from build123d import *

# Parameters (mm, degrees)
SKETCH_1_W          = 7.2
SKETCH_1_H          = 5
EXTRUDE_1_DEPTH     = 1.2
SKETCH_2_R          = 1.85
CUT_EXTRUDE_1_DEPTH = 5.544227107
SKETCH_3_W          = 1.2
SKETCH_3_H          = 5
EXTRUDE_2_DEPTH     = 24
FILLET_1_R          = 0.3
SKETCH_4_R          = 2.05
CUT_EXTRUDE_2_DEPTH = 27.024795869
EXTRUDE_START       = 2
EXTRUDE_4_DEPTH     = 2
EXTRUDE_5_DEPTH     = 1.2


with BuildPart() as part:
    # 스케치1 → 보스-돌출1 (new body)
    with BuildSketch(Plane.XY):
        Rectangle(SKETCH_1_W, SKETCH_1_H)
    extrude(amount=EXTRUDE_1_DEPTH)

    # 스케치2 → 컷-돌출1 (cut, through all)
    with BuildSketch(Plane.XY.offset(1.2)):
        with Locations((-0.75, 0)):
            Circle(SKETCH_2_R)
    extrude(amount=-CUT_EXTRUDE_1_DEPTH, mode=Mode.SUBTRACT)

    # 스케치3 → 보스-돌출2 (add)
    with BuildSketch(Plane.XY.offset(1.2)):
        with Locations((3, 0)):
            Rectangle(SKETCH_3_W, SKETCH_3_H)
    extrude(amount=EXTRUDE_2_DEPTH)

    # 필렛1
    fillet_1_edges = [part.edges().sort_by_distance(p)[0] for p in [
        (2.4, 0, 1.2),
    ]]
    fillet(fillet_1_edges, radius=FILLET_1_R)

    # 스케치4 → 컷-돌출2 (cut, through all)
    with BuildSketch(Plane.ZY.offset(-2.4)):
        with Locations(Location((21.2, 0, 0), (0, 0, 270))):
            Circle(SKETCH_4_R)
        with Locations(Location((9.2, 0, 0), (0, 0, 270))):
            Circle(SKETCH_4_R)
    extrude(amount=-CUT_EXTRUDE_2_DEPTH, mode=Mode.SUBTRACT)

    # 스케치6 → 보스-돌출4 (add)
    with BuildSketch(Plane.XZ.offset(2.5).offset(EXTRUDE_START)):
        with BuildLine():
            Line((-3.6, 1.2), (-3.6, 0))
            Line((-3.6, 0), (3.6, 0))
            Line((3.6, 0), (3.6, 25.2))
            Line((3.6, 25.2), (2.4, 25.2))
            Line((2.4, 25.2), (2.4, 1.5))
            ThreePointArc((2.4, 1.5), (2.312132034, 1.287867966), (2.1, 1.2))
            Line((2.1, 1.2), (-3.6, 1.2))
        make_face()
    extrude_4 = extrude(amount=-EXTRUDE_4_DEPTH)

    # 대칭 복사1: 보스-돌출4 across plane
    add(extrude_4.mirror(Plane.ZX))

    # 스케치7 → 보스-돌출5 (add)
    with BuildSketch(Plane(origin=(0, -4.5, 0), x_dir=(-1, 0, 0), z_dir=(0, -1, 0))):
        Polygon((3.6, 0), (-3.6, 0), (-3.6, -25.2), (-2.4, -25.2), (3.6, -1.2), align=None)
    extrude_5 = extrude(amount=EXTRUDE_5_DEPTH)

    # 대칭 복사2: 보스-돌출5 across plane
    add(extrude_5.mirror(Plane.ZX))


solid = part.part
Design review of the part built by this model. Coordinates are the model's own, in mm. A direction names the side the tool comes from. Give positions to 0.01 mm unless a question says otherwise; leave off trailing zeros. Loops run counter-clockwise (first coordinate to the right, second up) from the corner with the lowest first, then second, coordinate; pieces in that order, holes last. Notation, with made-up numbers: (-4.5, -35.75) - (41.5, -35.75) arc R16 cw to (41.5, -9.75) - close; hole circle Ø7 at (-31.5, 3.5). An arc over 180 degrees is marked (long way). Use CSV: the item, a comma, the result in double quotes. Start each with the question number.
1. Insertion check: P1, Ø4.5, axis at y = 2, z = 18.5, coming from the -X side; P2, Ø4, axis at x = -1, z = 18, coming from the +Y side. Each pin has a flat end and moves straight along its axis. Give the tip position at first contact, or say it passes through.
2. Add section B-B (z = 21.2). State the section outline as (x, y) points.
3. Add section A-A (x = -0.75). State the section outline as (y, z) points.
4. Draft analysis for pull direction Y (two halves, no side actions). For faces 3 (the flat face through (1, -1, 0)), 4 (the cylindrical face through (2.992, 0.444, 19.199)), 5 (the flat face through (1, -5.7, 10)), 6 (the cylindrical face through (2.992, -0.946, 7.381)), state which applies: released by +Y, released by -Y, zero draft, split by the parting line, or undercut.
5. Wall thickness on L1, parallel to Y at x = -0.75, z = 0.55; L2, parallel to Z at x = 3.15, y = 0; L3, parallel to X at y = -3, z = 6.25: over which ranges is each line inside the solid? List them lowest first.
6. Add section D-D (y = 4.25). State the section outline as (x, z) points, plus the area to 3 significant figures.
7. Machinability: for faces 1 (the flat face through (0, -4.5, 10)), 2 (the flat face through (3.6, 0, 12)), which of the approach directions +Z, -Z, +X, -X, +Y, -Y give a long, thin tool a straight path to every point of the face, cutting with its end or side? Answer none if there is none.
8. Add section C-C (x = 3). State the section outline as (y, z) points.
Results found:
1,P1,"stops at x = 2.4"
1,P2,"stops at y = 5.7"
2,outline,"(1.4, -5.7) - (3.6, -5.7) - (3.6, -2.05) - (2.4, -2.05) - (2.4, -4.5) - (1.4, -4.5) - close; (1.4, 4.5) - (2.4, 4.5) - (2.4, 2.05) - (3.6, 2.05) - (3.6, 5.7) - (1.4, 5.7) - close"
3,outline,"(-5.7, 0) - (-1.85, 0) - (-1.85, 1.2) - (-4.5, 1.2) - (-4.5, 12.6) - (-5.7, 12.6) - close; (1.85, 0) - (5.7, 0) - (5.7, 12.6) - (4.5, 12.6) - (4.5, 1.2) - (1.85, 1.2) - close"
4,face 3,"zero draft"
4,face 4,"undercut"
4,face 5,"released by -Y"
4,face 6,"undercut"
5,L1,"y = -5.7 to -1.85, 1.85 to 5.7"
5,L2,"z = 0 to 7.15, 11.25 to 19.15, 23.25 to 25.2"
5,L3,"x = 2.4 to 3.6"
6,outline,"(-3.6, 0) - (3.6, 0) - (3.6, 25.2) - (2.4, 25.2) - (2.4, 1.5) arc R0.3 cw to (2.1, 1.2) - (-3.6, 1.2) - close"
6,area,"37.5 mm²"
7,face 1,"+Z, -X"
7,face 2,"+Z, -Z, +X, +Y, -Y"
8,outline,"(-5.7, 0) - (5.7, 0) - (5.7, 25.2) - (-5.7, 25.2) - close; hole circle Ø4.1 at (0, 9.2); hole circle Ø4.1 at (0, 21.2)"
